Could you check a few things on this model? Use its own coordinates, in mm. Face numbers are marked on the shaded views. A direction names the side the tool comes from. Round coordinates to 2 decimals unless told otherwise and drop trailing zeros. Loops run counter-clockwise (first coordinate to the right, second up) from the corner with the lowest first, then second, coordinate; pieces in that order, holes last. Notation, with made-up numbers: (59.5, 25.5) -> (93.5, 25.5) arc R12 cw to (93.5, 46.5) -> close; hole circle Ø5 at (85.25, 43.5). An arc over 180 degrees is marked (long way). One line per item, written item: value.
```python
from build123d import *

# Parameters (mm, degrees)
F0_W      = 101.6
F0_H      = 76.2
F0_W_2    = 12.7
F0_H_2    = 63.5
F1_DEPTH  = 15.875
F2_R      = 5.08
F3_R      = 8.3185
F4_DEPTH  = 25.4
F5_DEPTH  = 66.675
F6_R      = 5.08
F7_R      = 12.7
F8_DEPTH  = 25.4
F9_W      = 6.35
F9_H      = 5.08
F10_DEPTH = 101.6


with BuildPart() as f1:
    # F0 (on Top) → F1 (new body)
    with BuildSketch(Plane.XY):
        Rectangle(F0_W, F0_H)
        Rectangle(F0_W_2, F0_H_2, mode=Mode.SUBTRACT)
    extrude(amount=F1_DEPTH)

    # F2
    f2_edges = [f1.edges().sort_by_distance(p)[0] for p in [
        (-50.8, 38.1, 7.9375),
        (-50.8, -38.1, 7.9375),
        (50.8, -38.1, 7.9375),
        (50.8, 38.1, 7.9375),
    ]]
    fillet(f2_edges, radius=F2_R)

    # F3 (on face) → F4 (cut)
    with BuildSketch(Plane.XY.offset(15.875)):
        with Locations((34.163, -21.463)):
            Circle(F3_R)
        with Locations((34.163, 21.463)):
            Circle(F3_R)
    extrude(amount=-F4_DEPTH, mode=Mode.SUBTRACT)

    # F0 (on Top) → F5 (join)
    with BuildSketch(Plane.XY):
        Rectangle(F0_W_2, F0_H_2)
    extrude(amount=F5_DEPTH)

    # F6
    f6_edges = [f1.edges().sort_by_distance(p)[0] for p in [
        (0, -31.75, 66.675),
        (0, 31.75, 66.675),
        (0, 31.75, 15.875),
        (0, -31.75, 15.875),
    ]]
    fillet(f6_edges, radius=F6_R)

    # F7 (on face) → F8 (cut)
    with BuildSketch(Plane(origin=(-6.35, 0, 0), x_dir=(0, -1, 0), z_dir=(-1, 0, 0))):
        with Locations((0, 41.275)):
            Circle(F7_R)
    extrude(amount=-F8_DEPTH, mode=Mode.SUBTRACT)

    # F9 (on face) → F10 (cut)
    with BuildSketch(Plane.XZ.offset(38.1)):
        with Locations((-25.4, 2.54)):
            Rectangle(F9_W, F9_H)
    extrude(amount=-F10_DEPTH, mode=Mode.SUBTRACT)


solid = f1.part
```
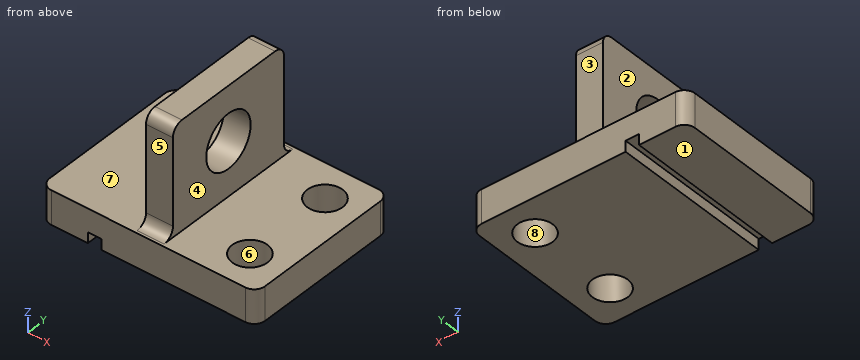
(1) Imagine slicing it at C-C on y = 0. Write out the boundary of the cut face in (x, z) (3 decimals).
Results below:
outline: (-50.8, 0) -> (-28.575, 0) -> (-28.575, 5.08) -> (-22.225, 5.08) -> (-22.225, 0) -> (50.8, 0) -> (50.8, 15.875) -> (6.35, 15.875) -> (6.35, 28.575) -> (-6.35, 28.575) -> (-6.35, 15.875) -> (-50.8, 15.875) -> close; (-6.35, 53.975) -> (6.35, 53.975) -> (6.35, 66.675) -> (-6.35, 66.675) -> close
(2) Imagine slicing it at B-B on z = 37. Write out the boundary of the cut face in (x, y), then the cut area to 3 significant figures.
Results below:
outline: (-6.35, -31.75) -> (6.35, -31.75) -> (6.35, -11.96) -> (-6.35, -11.96) -> close; (-6.35, 11.96) -> (6.35, 11.96) -> (6.35, 31.75) -> (-6.35, 31.75) -> close
area: 503 mm²
(3) Imagine slicing it at A-A on x = 40.5. Write out the boundary of the cut face in (y, z) (3 decimals).
Results below:
outline: (-38.1, 0) -> (-26.852, 0) -> (-26.852, 15.875) -> (-38.1, 15.875) -> close; (-16.074, 0) -> (16.074, 0) -> (16.074, 15.875) -> (-16.074, 15.875) -> close; (26.852, 0) -> (38.1, 0) -> (38.1, 15.875) -> (26.852, 15.875) -> close
(4) For pin 1 Ø8 at (y, z) = (-28.5, 27) entering from +X; pin 2 Ø8 at (x, z) = (-7.5, 39) entering from -Y; pin 3 Ø15 at (y, z) = (-4.5, 48.5) entering from -X, each with a flat end and sliding along its axis, tell me the tip position at first contact or that it passes through.
Results below:
pin 1: stops at x = 6.35
pin 2: stops at y = -31.75
pin 3: stops at x = -6.35
(5) On a 3-axis mill with a long thin cutter (end or side, diameter ignored), from which of +Z, -Z, +X, -X, +Y, -Y can I reach the whole of each face in a straight line? I mean the marked faces 1, 2, 3 and 4. Say none if no direction works.
Results below:
face 1: -Z, +X, -X, +Y, -Y
face 2: +Z, -X, +Y, -Y
face 3: +Z, +X, -X, +Y
face 4: +Z, +X, +Y, -Y
(6) Please list where these lines run through material, in increasing order: L1, parallel to X at y = 3, z = 3.5 (3 decimals); L2, parallel to X at y = 6.5, z = 19.5; L3, parallel to Z at x = -25, y = 28.5 (3 decimals).
Results below:
L1: x = -50.8 to -28.575, -22.225 to 50.8
L2: x = -6.35 to 6.35
L3: z = 5.08 to 15.875
(7) We'd pull the mould along Y, two halves only. Please class the marked faces 5, 6, 7 and 8: +Y half, -Y half, draft (parallel to the pull), parting line (faces both ways), or undercut.
Results below:
face 5: -Y half
face 6: undercut
face 7: draft
face 8: undercut
(8) Imagine slicing it at D-D on z = 8.5. Write out the boundary of the cut face in (x, y), then the cut area to 4 significant figures.
Results below:
outline: (-50.8, -33.02) arc R5.08 ccw to (-45.72, -38.1) -> (45.72, -38.1) arc R5.08 ccw to (50.8, -33.02) -> (50.8, 33.02) arc R5.08 ccw to (45.72, 38.1) -> (-45.72, 38.1) arc R5.08 ccw to (-50.8, 33.02) -> close; hole circle Ø16.64 at (34.16, -21.46); hole circle Ø16.64 at (34.16, 21.46)
area: 7,285 mm²
